The model under review builds one solid part; all positions refer to its coordinate system, in mm. A direction names the side the tool comes from. Round coordinates to 2 decimals unless told otherwise and drop trailing zeros. Order: outer loops, then holes, each group sorted by start corner. A loop starts at its lowest first (then second) coordinate and runs counter-clockwise, first axis right, second up. Notation, with made-up numbers: (-18.5, -14) -> (8.5, -14) arc R16 cw to (8.5, 11) -> close; hole circle Ø11 at (-30, 11). An arc over 180 degrees is marked (long way). Use a Markdown table: item, result. Add a question column.
```python
from build123d import *

# Parameters (mm, degrees)
FILLET_1_R = 5


with BuildPart() as part:
    # Эскиз1 → Повернуть1 (revolve)
    with BuildSketch(Plane(origin=(0, 0, 0), x_dir=(0, 0, -1), z_dir=(1, 0, 0))):
        Polygon((0, 50), (0, 20.5), (3, 20.5), (3, 47), (200, 47), (200, 50), align=None)
    revolve(axis=Axis((0, 0, 0), (0, 0, -1)))

    # Скругление1
    fillet_1_edges = [part.edges().sort_by_distance(p)[0] for p in [
        (0, -47, -3),
        (0, -50, 0),
    ]]
    fillet(fillet_1_edges, radius=FILLET_1_R)


solid = part.part
```
Q1. Insertion check: pin 1 (2 mm diameter, centred on x = -11, z = -85, fed in from -Y); pin 2 (2 mm diameter, centred on x = -12, z = -96.5, fed in from +Y) (3 decimals); pin 3 (4 mm diameter, centred on x = -39.5, z = -159, fed in from -Y); pin 4 (1.5 mm diameter, centred on x = -23, y = -25.5, fed in from +Z). Each pin has a flat end and moves straight along its axis. Give the tip position at first contact, or say it passes through.
Q2. Mouldability with a two-part tool opening along Y and no side actions: class faces 1 (the cylindrical face through (15.02, 47.69, -101.14)), 2 (the cylindrical face through (-20.013, -4.444, -1.521)), 3 (the flat face through (-19, 9, 0)) as pulls with the +Y half, pulls with the -Y half, needs draft (parallel to the pull), parting line crosses it, or undercut.
Q3. Machinability: for faces 4 (the flat face through (-33, 34, -200)), 5 (the cylindrical face through (14.12, 44.83, -105.34)), which of the approach directions +Z, -Z, +X, -X, +Y, -Y give a long, thin tool a straight path to every point of the face, cutting with its end or side? Answer none if there is none.
Q4. Wall thickness on line 1 (X direction, y = -1, z = -102); line 2 (Z direction, x = -1.5, y = -27); line 3 (Y direction, x = 23.5, z = -59): over which ranges is each line inside the solid? List them lowest first. Write a range as [from, to].
Q5. Add section B-B (z = -46). Write out the cut boundary in (x, y).
Q6. Add section A-A (y = 0). Write out the cut boundary in (x, z).
Report:
| question | item | result |
|---|---|---|
| 1 | pin 1 | stops at y = -48.99 |
| 1 | pin 2 | stops at y = 48.775 |
| 1 | pin 3 | stops at y = -33.07 |
| 1 | pin 4 | stops at z = 0 |
| 2 | face 1 | parting line crosses it |
| 2 | face 2 | undercut |
| 2 | face 3 | needs draft |
| 3 | face 4 | -Z, +X, -X, +Y, -Y |
| 3 | face 5 | -Z |
| 4 | line 1 | x = [-49.99, -46.99], [46.99, 49.99] |
| 4 | line 2 | z = [-3, 0] |
| 4 | line 3 | y = [-44.13, -40.7], [40.7, 44.13] |
| 5 | outline | circle Ø100 at (0, 0); hole circle Ø94 at (0, 0) |
| 6 | outline | (-50, -200) -> (-47, -200) -> (-47, -8) arc R5 cw to (-42, -3) -> (-20.5, -3) -> (-20.5, 0) -> (-45, 0) arc R5 ccw to (-50, -5) -> close; (20.5, -3) -> (42, -3) arc R5 cw to (47, -8) -> (47, -200) -> (50, -200) -> (50, -5) arc R5 ccw to (45, 0) -> (20.5, 0) -> close |
